from build123d import *

# Parameters (mm, degrees)
EXTRUDE_1_DEPTH = 4
FILLET_1_R      = 1.2


with BuildPart() as part:
    # 草图1 → 凸台-拉伸1 (new body)
    with BuildSketch(Plane.XY):
        Polygon((14.909090909, 14), (14.909090909, -96), (6.909090909, -96), (6.909090909, -91), (-2.590909091, -91), (-2.590909091, -87), (-1.290909091, -87), (-1.290909091, -84.5), (-2.590909091, -84.5), (-2.590909091, -82), (-5.590909091, -82), (-5.590909091, -84.5), (-6.890909091, -84.5), (-6.890909091, -87), (-5.590909091, -87), (-5.590909091, -91), (-15.090909091, -91), (-15.090909091, -96), (-23.090909091, -96), (-23.090909091, 14), (-15.090909091, 14), (-15.090909091, 9), (-5.590909091, 9), (-5.590909091, 5), (-6.890909091, 5), (-6.890909091, 2.5), (-5.590909091, 2.5), (-5.590909091, 0), (-2.590909091, 0), (-2.590909091, 2.5), (-1.290909091, 2.5), (-1.290909091, 5), (-2.590909091, 5), (-2.590909091, 9), (6.909090909, 9), (6.909090909, 14), align=None)
    extrude(amount=EXTRUDE_1_DEPTH)

    # 圆角1
    fillet_1_edges = [part.edges().sort_by_distance(p)[0] for p in [
        (6.909090909, 14, 2),
        (14.909090909, 14, 2),
        (14.909090909, -96, 2),
        (6.909090909, -96, 2),
        (-15.090909091, -96, 2),
        (-23.090909091, -96, 2),
        (-23.090909091, 14, 2),
        (-15.090909091, 14, 2),
    ]]
    fillet(fillet_1_edges, radius=FILLET_1_R)


solid = part.part
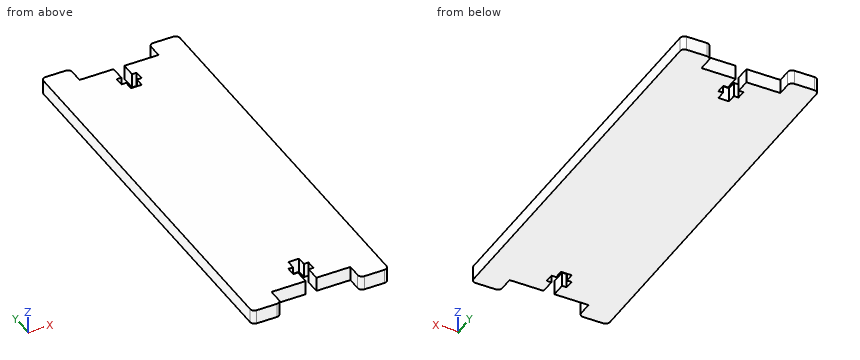
Model file for the job. Use its own axes, mm. Give positions to 0.01 mm unless a question says otherwise; leave off trailing zeros. Loops run counter-clockwise (first coordinate to the right, second up) from the corner with the lowest first, then second, coordinate; pieces in that order, holes last.
1) Saw through at A-A (y = -85.5). Write the cut outline in (x, z), plus the area to 3 significant figures.
2) Wall check: line 1 (X direction, y = 7, z = 1.7); line 2 (Y direction, x = -12.5, z = 2.95); line 3 (Y direction, x = -4, z = 0.6). Give the ranges that are in metal, low to high.
3) Saw through at B-B (x = -11). Write the cut outline in (y, z), plus the area to 3 significant figures.
4) Flat gauge pins, fed straight in: pin 1 Ø0.6 at (x, z) = (-6.5, 2) entering from +Y; pin 2 Ø2 at (x, z) = (-12.5, 2) entering from -Y. Where does each tip first touch, or does it go through?
Answer block:
1. outline: (-23.09, 0) - (-6.89, 0) - (-6.89, 4) - (-23.09, 4) - close; (-1.29, 0) - (14.91, 0) - (14.91, 4) - (-1.29, 4) - close
1. area: 130 mm2
2. line 1: x = -23.09 to -5.59, -2.59 to 14.91
2. line 2: y = -91 to 9
2. line 3: y = -82 to 0
3. outline: (-91, 0) - (9, 0) - (9, 4) - (-91, 4) - close
3. area: 400 mm2
4. pin 1: stops at y = 9
4. pin 2: stops at y = -91
